The listing builds one solid part. Answer for the finished solid, in the listing's coordinates (mm). A direction names the side the tool comes from. Coordinates: 2 decimals unless noted, no trailing zeros. Loops run counter-clockwise (first coordinate to the right, second up) from the corner with the lowest first, then second, coordinate; pieces in that order, holes last. Notation, with made-up numbers: (49, 68) - (62, 68) arc R9 ccw to (62, 82) - close; hole circle Ø2 at (11.25, -36). An arc over 180 degrees is marked (long way). Return JSON: item names as keys, results as strings. Group by question number.
1. Find the intervals of material crossed by line 1 along Z through (x, y) = (-85.5, 0); line 2 along X through (y, z) = (-11.5, -13); line 3 along Z through (x, y) = (-68.5, -1), in increasing order.
2. Section A-A (x = -28.5) is taken. Write down the section's boundary in (y, z), and give its area (3 significant figures).
3. The mould has two halves that part along Z. Classify faces 4 (the face through (85.619, 11.923, 3.755)), 5 (the face through (95, 0, 0)), 6 (the face through (-77.89, -0.72, -0.16)): pulls with the +Z half, pulls with the -Z half, needs draft (parallel to the pull), parting line crosses it, or undercut.
4. Section B-B (x = -59) is taken. Write down the section's boundary in (y, z).
5. Which of the six approach directions +Z, -Z, +X, -X, +Y, -Y give full straight-line access (tool end or side, diameter ignored) to faces 1 (the face through (75, 2.8, 14.4)), 2 (the face through (-80.311, -14.985, 0.66)), 3 (the face through (0, 0, -27))?
6. Each of these flat-tipped pins is pushed along its axis until it touches: P1, Ø10, axis at x = -14.5, y = 7, coming from the +Z side; P2, Ø18, axis at y = -5, z = 11, coming from the +X side; P3, Ø1.5, axis at x = -20.5, z = 10.5, coming from the +Y side; P4, Ø2, axis at x = 54.5, y = 13, coming from the -Z side. Where does it stop, or does it pass through?
```python
from build123d import *

# Parameters (mm, degrees)
CHANFRO1_SIZE                    = 1
FILETE1_R                        = 2
FURO_ROSCADO_DE_M101_D           = 8.5
FURO_ROSCADO_DE_M101_DEPTH       = 15
FURO_ROSCADO_DE_M101_CSINK_D     = 10.05
FURO_ROSCADO_DE_M101_CSINK_ANGLE = 90
FURO_ROSCADO_DE_M101_TIP         = 2.553657631


with BuildPart() as part:
    # Esboço1 → Revolução1 (revolve)
    with BuildSketch(Plane.XY):
        with BuildLine():
            Line((-95, 0), (-95, 15))
            Line((-95, 15), (-65, 15))
            Line((-65, 15), (-65, 19.420381157))
            Line((-65, 19.420381157), (-5, 30))
            Line((-5, 30), (0, 30))
            Line((0, 30), (0, 26.519237886))
            ThreePointArc((0, 26.519237886), (15, 22.5), (30, 26.519237886))
            Line((30, 26.519237886), (30, 30))
            Line((30, 30), (35, 30))
            Line((35, 30), (75, 19.282032303))
            Line((75, 19.282032303), (75, 12.5))
            Line((75, 12.5), (95, 12.5))
            Line((95, 12.5), (95, 0))
            Line((95, 0), (-95, 0))
        make_face()
    revolve(axis=Axis((-95, 0, 0), (1, 0, 0)))

    # Chanfro1
    chanfro1_edges = [part.edges().sort_by_distance(p)[0] for p in [
        (-95, -15, 0),
        (95, -12.5, 0),
    ]]
    chamfer(chanfro1_edges, length=CHANFRO1_SIZE)

    # Filete1
    filete1_edges = [part.edges().sort_by_distance(p)[0] for p in [
        (-65, -15, 0),
        (75, -12.5, 0),
    ]]
    fillet(filete1_edges, radius=FILETE1_R)

    # Furo roscado de M101
    with Locations(Plane.ZY.offset(95)):
        with Locations((0, 0)):
            CounterSinkHole(FURO_ROSCADO_DE_M101_D / 2, FURO_ROSCADO_DE_M101_CSINK_D / 2, depth=FURO_ROSCADO_DE_M101_DEPTH, counter_sink_angle=FURO_ROSCADO_DE_M101_CSINK_ANGLE)
            with Locations((0, 0, -(FURO_ROSCADO_DE_M101_DEPTH + FURO_ROSCADO_DE_M101_TIP / 2))):  # 118° drill point
                Cone(0, FURO_ROSCADO_DE_M101_D / 2, FURO_ROSCADO_DE_M101_TIP, mode=Mode.SUBTRACT)


solid = part.part
```
The answers:
{
 "1": {"line 1": "z = -15 to -4.25, 4.25 to 15", "line 2": "x = -65 to 75", "line 3": "z = -14.97 to 14.97"},
 "2": {"outline": "circle Ø51.71 at (0, 0)", "area": "2,100 mm2"},
 "3": {"face 4": "parting line crosses it", "face 5": "needs draft", "face 6": "undercut"},
 "4": {"outline": "circle Ø40.96 at (0, 0)"},
 "5": {"face 1": "+X", "face 2": "-X", "face 3": "none"},
 "6": {"P1": "stops at z = 28.75", "P2": "stops at x = 95", "P3": "stops at y = 25.5", "P4": "stops at z = -21.75"}
}
